CAD build for the part. Positions are in the model's coordinates, mm. A direction names the side the tool comes from. Round coordinates to 2 decimals unless told otherwise and drop trailing zeros. Write each loop counter-clockwise with the first axis right and the second up, starting at its lowest first coordinate (ties: lowest second). Pieces come first, ordered by that corner, then holes. Notation, with made-up numbers: (17.25, 60.5) - (49.25, 60.5) arc R18 ccw to (49.25, 77.5) - close; hole circle Ø7 at (69.25, -3.75). An arc over 180 degrees is marked (long way). Answer in a Markdown table with one row per item.
Autodesk Inventor part; units mm, degrees
ref_plane "Work Plane1" through (0, 0, 30) normal (0, 0, 1) x (1, 0, 0)
ref_plane "YZ Plane" through (0, 0, 0) normal (1, 0, 0) x (0, 1, 0)
ref_plane "XZ Plane" through (0, 0, 0) normal (0, 1, 0) x (-1, 0, 0)
sketch "Sketch1" plane through (0, 0, 0) normal (0, 0, 1) x (1, 0, 0)
  circle A0 centre (20, 109) radius 11
  circle A1 centre (20, 20) radius 13
  line L0 (20, 109) -> (20, 20) construction
  line L1 (0, 144) -> (0, -24) construction
  line L2 (-16.8865, 0) -> (101.3193, 0) construction
  circle A2 centre (30, 60) radius 24
  line L3 (23.5359, 84.7724) -> (16.2342, 79.6596)
  line L4 (10.9893, 102.6907) -> (23.5359, 84.7724)
  line L5 (30, 60) -> (20, 20) construction
  line L6 (15.0071, 41.2593) -> (12.3132, 30.484)
  line L7 (34.4099, 36.4086) -> (31.7161, 25.6333)
  line L8 (29.0107, 115.3093) -> (35.8214, 105.5826)
  line L9 (35.8214, 105.5826) -> (44.2824, 111.507)
  line L10 (44.2824, 111.507) -> (84.4327, 54.1663)
  line L11 (84.4327, 54.1663) -> (38.1631, 37.4309)
  circle A3 centre (69.6897, 31.6354) radius 7.5
  line L12 (84.4327, 54.1663) -> (76.861, 29.4394)
  line L13 (62.6369, 29.0844) -> (57.1359, 44.2933)
  point P0 (0, 0)
  dimension "d0" = 89
  dimension "d2" = 48
  dimension "d3" = 20
  dimension "d4" = 20
  dimension "d5" = 26
  dimension "d6" = 22
  dimension "d7" = 40
  dimension "d8" = 10
  dimension "d9" = 35
  dimension "d10" = 20
  dimension "d11" = 10
  dimension "d13" = 10.3289
  dimension "d14" = 70
  dimension "d15" = 25
  dimension "d17" = 80
  dimension "d18" = 15
extrude "Extrusion1" add sketch "Sketch1" against normal blind 38
ref_plane "Work Plane1" through (0, 0, 30) normal (0, 0, 1) x (1, 0, 0)
sketch "Sketch2" plane through (0, 0, 30) normal (0, 0, 1) x (1, 0, 0)
  line L0 (10.9893, 102.6907) -> (23.5359, 84.7724)
  line L1 (23.5359, 84.7724) -> (16.2342, 79.6596)
  arc A0 (16.2342, 79.6596) -> (15.0071, 41.2593) centre (30, 60) ccw
  line L2 (15.0071, 41.2593) -> (12.3132, 30.484)
  arc A1 (12.3132, 30.484) -> (31.7161, 25.6333) centre (20, 20) ccw
  line L3 (31.7161, 25.6333) -> (34.4099, 36.4086)
  arc A2 (34.4099, 36.4086) -> (38.1631, 37.4309) centre (30, 60) ccw
  line L4 (38.1631, 37.4309) -> (57.1359, 44.2933)
  line L5 (57.1359, 44.2933) -> (62.6369, 29.0844)
  arc A3 (62.6369, 29.0844) -> (76.861, 29.4394) centre (69.6897, 31.6354) ccw
  line L6 (76.861, 29.4394) -> (84.4327, 54.1663)
  line L7 (84.4327, 54.1663) -> (44.2824, 111.507)
  arc A4 (29.0107, 115.3093) -> (10.9893, 102.6907) centre (20, 109) ccw
  line L8 (84.4327, 54.1663) -> (36.9219, 20.8989)
  line L9 (44.2824, 111.507) -> (-3.2284, 78.2395)
  line L10 (35.8214, 105.5826) -> (29.0107, 115.3093)
  line L11 (-3.2284, 78.2395) -> (2.5073, 70.048)
  line L12 (36.9219, 20.8989) -> (31.1862, 29.0904)
  line L13 (2.5073, 70.048) -> (31.1862, 29.0904) construction
  circle A5 centre (41.4213, 66.7765) radius 20
  line L14 (41.4213, 66.7765) -> (16.8468, 49.5692) construction
  line L15 (2.5073, 70.048) -> (32.6535, 84.7522)
  line L16 (31.1862, 29.0904) -> (55.3141, 52.3894)
  point P0 (0, 0)
  point P1 (17.8001, 92.9639)
  point P2 (33.0241, 30.8652)
  point P3 (32.2136, 27.6232)
  point P4 (59.8027, 36.9202)
  dimension "d23" = 58
  dimension "d27" = 10
  dimension "d28" = 30
  dimension "d29" = 40
extrude "Extrusion2" add sketch "Sketch2" along normal blind 17 contours A4 L10 L9 L0 | L9 L7 L8 L5 L4 L16 A5 L15 A0 L1 L0 | L0 L1 A0 L15 L11 L9 | L6 A3 L5 L8 | L8 L12 L3 L16 L4 L5
sketch "Sketch3" plane through (0, 0, 30) normal (0, 0, -1) x (-1, 0, 0)
  line L0 (-10.9893, 102.6907) -> (-17.8001, 92.9639)
  arc A0 (-10.9893, 102.6907) -> (-29.0107, 115.3093) centre (-20, 109) ccw
  line L1 (-35.8214, 105.5826) -> (-29.0107, 115.3093)
  line L2 (-44.2824, 111.507) -> (-35.8214, 105.5826)
  line L3 (-84.4327, 54.1663) -> (-44.2824, 111.507)
  line L4 (-76.861, 29.4394) -> (-84.4327, 54.1663)
  arc A1 (-76.861, 29.4394) -> (-62.6369, 29.0844) centre (-69.6897, 31.6354) ccw
  line L5 (-59.8027, 36.9202) -> (-62.6369, 29.0844)
  line L6 (-36.9219, 20.8989) -> (-59.8027, 36.9202)
  line L7 (-32.2136, 27.6232) -> (-36.9219, 20.8989)
  line L8 (-33.0241, 30.8652) -> (-32.2136, 27.6232)
  line L9 (-55.3141, 52.3894) -> (-33.0241, 30.8652)
  arc A2 (-32.6535, 84.7522) -> (-55.3141, 52.3894) centre (-41.4213, 66.7765) ccw
  line L10 (-2.5073, 70.048) -> (-32.6535, 84.7522)
  line L11 (3.2284, 78.2395) -> (-2.5073, 70.048)
  line L12 (-17.8001, 92.9639) -> (3.2284, 78.2395)
  line L13 (-59.8027, 36.9202) -> (-84.4327, 54.1663)
  line L14 (-35.8214, 105.5826) -> (-17.8001, 92.9639)
  line L15 (-27.8994, 100.0354) -> (-37.4607, 86.3804)
  line L16 (-84.4327, 54.1663) -> (-44.2824, 111.507)
  line L17 (-68.0497, 42.6948) -> (-58.4884, 56.3498)
  line L18 (-32.493, 93.475) -> (-48.8761, 104.9465) construction
  line L19 (-63.269, 49.5223) -> (-79.6521, 60.9938) construction
  point P0 (0, 0)
  dimension "d52" = 20
extrude "Extrusion3" add sketch "Sketch3" along normal up to surface (30 mm away) contours L15 A2 L17 L13 L3 L2 L14
sketch "Sketch4" plane through (0, 0, 0) normal (0, 0, 1) x (1, 0, 0)
  arc A0 (29.0107, 115.3093) -> (10.9893, 102.6907) centre (20, 109) ccw
  point P0 (0, 0)
hole "Hole1" at (20, 109, 0) direction (0, 0, -1) diameter 8.376 end through all
sketch "Sketch5" plane through (0, 0, 0) normal (0, 0, 1) x (1, 0, 0)
  arc A0 (12.3132, 30.484) -> (31.7161, 25.6333) centre (20, 20) ccw
  point P0 (0, 0)
hole "Hole2" at (20, 20, 0) direction (0, 0, -1) diameter 6 end through all
sketch "Sketch6" plane through (0, 0, 0) normal (0, 0, 1) x (1, 0, 0)
  circle A0 centre (20, 20) radius 3
  circle A1 centre (20, 109) radius 4.188
  arc A2 (58.4884, 56.3498) -> (37.4607, 86.3804) centre (41.4213, 66.7765) ccw
  line L0 (27.8994, 100.0354) -> (35.8214, 105.5826)
  line L1 (35.8214, 105.5826) -> (29.0107, 115.3093)
  arc A3 (29.0107, 115.3093) -> (10.9893, 102.6907) centre (20, 109) ccw
  line L2 (10.9893, 102.6907) -> (23.5359, 84.7724)
  arc A4 (16.2342, 79.6596) -> (15.0071, 41.2593) centre (30, 60) ccw
  line L3 (15.0071, 41.2593) -> (12.3132, 30.484)
  arc A5 (12.3132, 30.484) -> (31.7161, 25.6333) centre (20, 20) ccw
  line L4 (31.7161, 25.6333) -> (34.4099, 36.4086)
  arc A6 (34.4099, 36.4086) -> (38.1631, 37.4309) centre (30, 60) ccw
  line L5 (38.1631, 37.4309) -> (57.1359, 44.2933)
  line L6 (34.4099, 36.4086) -> (15.0071, 41.2593)
  line L7 (84.4327, 54.1663) -> (68.0497, 42.6948)
  line L8 (68.0497, 42.6948) -> (58.4884, 56.3498)
  line L9 (37.4607, 86.3804) -> (27.8994, 100.0354)
  line L10 (23.5359, 84.7724) -> (16.2342, 79.6596)
  line L11 (57.1359, 44.2933) -> (62.6369, 29.0844)
  arc A7 (62.6369, 29.0844) -> (76.861, 29.4394) centre (69.6897, 31.6354) ccw
  line L12 (76.861, 29.4394) -> (84.4327, 54.1663)
  point P0 (0, 0)
extrude "Extrusion4" cut sketch "Sketch6" against normal blind 10 contours L4 A5 L3 L6
sketch "Sketch7" plane through (0, 0, 0) normal (0, 0, 1) x (1, 0, 0)
  line L0 (15.0071, 41.2593) -> (34.4099, 36.4086)
  arc A0 (34.4099, 36.4086) -> (38.1631, 37.4309) centre (30, 60) ccw
  line L1 (38.1631, 37.4309) -> (57.1359, 44.2933)
  arc A1 (58.4884, 56.3498) -> (37.4607, 86.3804) centre (41.4213, 66.7765) ccw
  line L2 (27.8994, 100.0354) -> (35.8214, 105.5826)
  line L3 (35.8214, 105.5826) -> (29.0107, 115.3093)
  arc A2 (29.0107, 115.3093) -> (10.9893, 102.6907) centre (20, 109) ccw
  line L4 (10.9893, 102.6907) -> (23.5359, 84.7724)
  arc A3 (16.2342, 79.6596) -> (15.0071, 41.2593) centre (30, 60) ccw
  circle A4 centre (20, 109) radius 4.188
  line L5 (19.6524, 94.2609) -> (17.2626, 93.7315)
  line L6 (57.1359, 44.2933) -> (62.6369, 29.0844)
  arc A5 (62.6369, 29.0844) -> (76.861, 29.4394) centre (69.6897, 31.6354) ccw
  line L7 (76.861, 29.4394) -> (84.4327, 54.1663)
  line L8 (84.4327, 54.1663) -> (68.0497, 42.6948)
  line L9 (68.0497, 42.6948) -> (58.4884, 56.3498)
  line L10 (37.4607, 86.3804) -> (27.8994, 100.0354)
  line L11 (23.5359, 84.7724) -> (16.2342, 79.6596)
  point P0 (0, 0)
extrude "Extrusion5" cut sketch "Sketch7" against normal blind 6.5
properties part number "F3_Rough_Rear_Caliper_V2"
Q1. Pull direction Z, two halves, no side cores. Call faces 6 (the cylindrical face through (13.89, 118.147, -22.03)), 7 (the flat face through (21, 24, -10)), 8 (the flat face through (21, 95, 30)): released by +Z, released by -Z, zero draft, split by the parting line, or undercut.
Computed:
| item | result |
|---|---|
| face 6 | zero draft |
| face 7 | released by +Z |
| face 8 | undercut |
Q2. Saw through at A-A on y = 109. List the corners of the cut face in (x, z).
Computed:
| item | result |
|---|---|
| outline | (9, -38) - (15.81, -38) - (15.81, -6.5) - (9, -6.5) - close; (9, 30) - (33.43, 30) - (33.43, 47) - (9, 47) - close; (24.19, -38) - (33.43, -38) - (33.43, -6.5) - (24.19, -6.5) - close; (40.7, -38) - (46.04, -38) - (46.04, 47) - (40.7, 47) - close |
Q3. Flat gauge pins, fed straight in: pin 1 (1 mm diameter, centred on x = 19.5, y = 58, fed in from +Z); pin 2 (7 mm diameter, centred on x = 20, y = 20, fed in from -Z); pin 3 (1.5 mm diameter, centred on y = 94.5, z = 18.5, fed in from -X); pin 4 (2 mm diameter, centred on y = 57, z = 30, fed in from +X). Where does each tip first touch, or does it go through?
Computed:
| item | result |
|---|---|
| pin 1 | stops at z = -6.5 |
| pin 2 | stops at z = -38 |
| pin 3 | stops at x = 31.25 |
| pin 4 | stops at x = 83.15 |
Q4. Saw through at C-C on z = 38. List the corners of the cut face in (x, y), then the cut area to 3 significant figures.
Computed:
| item | result |
|---|---|
| outline | (-3.23, 78.24) - (2.51, 70.05) - (32.65, 84.75) arc R20 cw to (55.31, 52.39) - (33.02, 30.87) - (32.21, 27.62) - (36.92, 20.9) - (59.8, 36.92) - (62.64, 29.08) arc R7.5 ccw to (76.86, 29.44) - (84.43, 54.17) - (44.28, 111.51) - (35.82, 105.58) - (29.01, 115.31) arc R11 ccw to (10.99, 102.69) - (17.8, 92.96) - close |
| area | 2,870 mm2 |
Q5. Drill centre lines: line 1 (X direction, y = 20, z = -29.25); line 2 (Y direction, x = 20, z = -29); line 3 (X direction, y = 109, z = -18). Where is each one in solid material? Low to high.
Computed:
| item | result |
|---|---|
| line 1 | x = 7 to 17, 23 to 33 |
| line 2 | y = 7 to 17, 23 to 82.3, 89.82 to 104.81, 113.19 to 120 |
| line 3 | x = 9 to 15.81, 24.19 to 33.43, 40.7 to 46.04 |
Q6. Saw through at B-B on x = 20. List the corners of the cut face in (y, z).
Computed:
| item | result |
|---|---|
| outline | (7, -38) - (17, -38) - (17, -10) - (7, -10) - close; (23, -38) - (82.3, -38) - (82.3, -6.5) - (40.01, -6.5) - (40.01, -10) - (23, -10) - close; (78.58, 30) - (120, 30) - (120, 47) - (78.58, 47) - close; (89.82, -38) - (104.81, -38) - (104.81, -6.5) - (89.82, -6.5) - close; (113.19, -38) - (120, -38) - (120, -6.5) - (113.19, -6.5) - close |
Q7. 3-axis set-ups, long thin cutter, end or side, ignore diameter. For faces 1 (the flat face through (32.46, 110.38, 38.38)), 2 (the flat face through (63.336, 49.427, 12.006)), 3 (the flat face through (59.925, 36.582, -22.03)), 4 (the flat face through (24.84, 38.8, -8.23)), 5 (the flat face through (7.433, 85.705, 38.381)): which of +Z, -Z, +X, -X, +Y, -Y reach the whole face in a straight line?
Computed:
| item | result |
|---|---|
| face 1 | +Z, -Z, +Y |
| face 2 | -X, -Y |
| face 3 | -Z, -Y |
| face 4 | +Z, -X, -Y |
| face 5 | +Z, -Z, -X |
Q8. Saw through at D-D on z = -24. List the corners of the cut face in (x, y), then the cut area to 3 significant figures.
Computed:
| item | result |
|---|---|
| outline | (10.99, 102.69) - (23.54, 84.77) - (16.23, 79.66) arc R24 ccw to (15.01, 41.26) - (12.31, 30.48) arc R13 ccw (long way) to (31.72, 25.63) - (34.41, 36.41) arc R24 ccw to (38.16, 37.43) - (57.14, 44.29) - (62.64, 29.08) arc R7.5 ccw to (76.86, 29.44) - (84.43, 54.17) - (44.28, 111.51) - (35.82, 105.58) - (29.01, 115.31) arc R11 ccw to start; hole circle Ø8.38 at (20, 109); hole circle Ø6 at (20, 20) |
| area | 4,960 mm2 |
